```python
from build123d import *

# Parameters (mm, degrees)
F0_R     = 0.75
F0_W     = 85
F0_H     = 45
F1_DEPTH = 2


with BuildPart() as f1:
    # F0 (on Top) → F1 (new body)
    with BuildSketch(Plane.XY):
        with BuildLine():
            ThreePointArc((55, 32), (54.12132, 34.12132), (52, 35))
            Line((52, 35), (-52, 35))
            ThreePointArc((-52, 35), (-54.12132, 34.12132), (-55, 32))
            Line((-55, 32), (-55, -32))
            ThreePointArc((-55, -32), (-54.12132, -34.12132), (-52, -35))
            Line((-52, -35), (52, -35))
            ThreePointArc((52, -35), (54.12132, -34.12132), (55, -32))
            Line((55, -32), (55, 32))
        make_face()
        with Locations((-51.3, -31.3)):
            Circle(F0_R, mode=Mode.SUBTRACT)
        with Locations((51.3, -31.3)):
            Circle(F0_R, mode=Mode.SUBTRACT)
        with Locations((-51.3, 31.3)):
            Circle(F0_R, mode=Mode.SUBTRACT)
        Rectangle(F0_W, F0_H, mode=Mode.SUBTRACT)
        with Locations((51.3, 31.3)):
            Circle(F0_R, mode=Mode.SUBTRACT)
    extrude(amount=F1_DEPTH)


solid = f1.part
```
Verification items for the finished model (mm, model axes). A direction names the side the tool comes from. Coordinates: 2 decimals unless noted, no trailing zeros. Order: outer loops, then holes, each group sorted by start corner. A loop starts at its lowest first (then second) coordinate and runs counter-clockwise, first axis right, second up. Notation, with made-up numbers: (60, 77.5) -> (108, 77.5) arc R20 ccw to (108, 100.5) -> close; hole circle Ø1 at (58, 30). An arc over 180 degrees is marked (long way). Put each result on its own line as item: value. Start each with the question number.
1) Tool access check on faces 4 (the cylindrical face through (54.1, -34.14, 0.99)), 5 (the flat face through (-42.5, 0, 1)). Record the directions out of +Z, -Z, +X, -X, +Y, -Y that give a thin tool (end or side, any length) a straight path to the whole face; none if there is none.
2) Cross-section at C-C (x = -13.5). Enter the section's corners in (y, z), plus the area to 3 significant figures.
3) Cross-section at B-B (z = 0.4). Enter the section's corners in (x, y).
4) Cross-section at A-A (y = -2.5). Enter the section's corners in (x, z).
5) Release check for a two-part mould opening along Y. For faces 1 (the flat face through (-1, 22.5, 1)), 2 (the cylindrical face through (-54.14, -34.1, 0.99)), 3 (the flat face through (1, 35, 1)) record: pulls with the +Y half, pulls with the -Y half, needs draft (parallel to the pull), parting line crosses it, or undercut.
6) Go/stop test with a flat-tipped pin: pin 1 (1.7 mm diameter, centred on x = 51.3, y = -31.3, fed in from +Z). Record where the tip stops, or that it passes through.
7) Material ranges on L1, parallel to Y at x = -51.3, z = 0.4; L2, parallel to X at y = -19, z = 1.7; L3, parallel to Y at x = 25.5, z = 1.45, recorded low to high.
Geometry check:
1. face 4: +Z, -Z, +X, -Y
1. face 5: +Z, -Z
2. outline: (-35, 0) -> (-22.5, 0) -> (-22.5, 2) -> (-35, 2) -> close; (22.5, 0) -> (35, 0) -> (35, 2) -> (22.5, 2) -> close
2. area: 50.0 mm^2
3. outline: (-55, -32) arc R3 ccw to (-52, -35) -> (52, -35) arc R3 ccw to (55, -32) -> (55, 32) arc R3 ccw to (52, 35) -> (-52, 35) arc R3 ccw to (-55, 32) -> close; hole circle Ø1.5 at (-51.3, -31.3); hole circle Ø1.5 at (-51.3, 31.3); hole (-42.5, -22.5) -> (42.5, -22.5) -> (42.5, 22.5) -> (-42.5, 22.5) -> close; hole circle Ø1.5 at (51.3, -31.3); hole circle Ø1.5 at (51.3, 31.3)
4. outline: (-55, 0) -> (-42.5, 0) -> (-42.5, 2) -> (-55, 2) -> close; (42.5, 0) -> (55, 0) -> (55, 2) -> (42.5, 2) -> close
5. face 1: undercut
5. face 2: pulls with the -Y half
5. face 3: pulls with the +Y half
6. pin 1: stops at z = 2
7. L1: y = -35 to -32.05, -30.55 to 30.55, 32.05 to 35
7. L2: x = -55 to -42.5, 42.5 to 55
7. L3: y = -35 to -22.5, 22.5 to 35
